For this review, take the finished solid that the model builds, in its own axes (mm). A direction names the side the tool comes from. Give positions to 0.01 mm unless a question says otherwise; leave off trailing zeros. Write each loop counter-clockwise with the first axis right and the second up, starting at its lowest first coordinate (ties: lowest second). Pieces come first, ordered by that corner, then holes.
from build123d import *

# Parameters (mm, degrees)
SKETCH1_W                = 50
SKETCH1_H                = 50
BOSS_EXTRUDE1_DEPTH      = 50
CHAMFER1_SIZE            = 1.5
BOSS_EXTRUDE2_DEPTH      = 7
BOSS_EXTRUDE2_DEPTH_BACK = 7
SKETCH6_W                = 1
SKETCH6_H                = 7
SKETCH7_W                = 1.8
SKETCH7_H                = 1.8
CUT_EXTRUDE1_DEPTH       = 7


with BuildPart() as part:
    # Sketch1 → Boss-Extrude1 (new body)
    with BuildSketch(Plane.XY):
        with Locations((25, 25)):
            Rectangle(SKETCH1_W, SKETCH1_H)
    extrude(amount=BOSS_EXTRUDE1_DEPTH)

    # Cut-Sweep2: sweep along a path in Sketch4
    with BuildLine(Plane.XY.offset(50)) as cut_sweep2_path:
        Line((25, 50), (25, 47))
        ThreePointArc((25, 47), (31.443650814, 31.443650814), (47, 25))
        Line((47, 25), (50, 25))
    # Sketch3 → Cut-Sweep2 (sweep, cut)
    with BuildSketch(Plane.XZ.offset(-50)):
        Polygon((29.556349186, 39), (36, 45.443650814), (36, 54.556349186), (29.556349186, 61), (20.443650814, 61), (14, 54.556349186), (14, 45.443650814), (20.443650814, 39), align=None)
    sweep(path=cut_sweep2_path.line, mode=Mode.SUBTRACT)

    # Sketch5 → Cut-Loft1 section 0
    with BuildSketch(Plane.ZY):
        with BuildLine():
            Line((24.5, 20.443650814), (24.5, 29.556349186))
            Line((24.5, 29.556349186), (18.056349186, 36))
            Line((18.056349186, 36), (8.943650814, 36))
            Line((8.943650814, 36), (2.5, 29.556349186))
            Line((2.5, 29.556349186), (2.5, 20.443650814))
            Line((2.5, 20.443650814), (8.943650814, 14))
            Line((8.943650814, 14), (18.056349186, 14))
            Line((18.056349186, 14), (24.5, 20.443650814))
        make_face()
    # Sketch2 → Cut-Loft1 section 1
    with BuildSketch(Plane.ZY.offset(-50)):
        with BuildLine():
            Line((36, 29.556349186), (29.556349186, 36))
            Line((29.556349186, 36), (20.443650814, 36))
            Line((20.443650814, 36), (14, 29.556349186))
            Line((14, 29.556349186), (14, 20.443650814))
            Line((14, 20.443650814), (20.443650814, 14))
            Line((20.443650814, 14), (29.556349186, 14))
            Line((29.556349186, 14), (36, 20.443650814))
            Line((36, 20.443650814), (36, 29.556349186))
        make_face()
    loft(mode=Mode.SUBTRACT)

    # Chamfer1
    chamfer1_edges = [part.edges().sort_by_distance(p)[0] for p in [
        (50, 7, 50),
        (43, 50, 50),
        (50, 43, 50),
        (7, 50, 50),
        (14, 48.5, 50),
        (23.665476221, 23.665476221, 50),
        (48.5, 14, 50),
        (36, 48.5, 50),
        (39.221825407, 39.221825407, 50),
        (48.5, 36, 50),
        (36, 50, 47.721825407),
        (14, 50, 47.721825407),
        (50, 36, 47.721825407),
        (50, 14, 47.721825407),
        (50, 17.221825407, 42.221825407),
        (50, 32.778174593, 42.221825407),
        (32.778174593, 50, 42.221825407),
        (17.221825407, 50, 42.221825407),
        (0, 25, 50),
        (25, 50, 0),
        (50, 25, 0),
        (25, 0, 0),
        (0, 25, 0),
        (25, 0, 50),
        (0, 50, 25),
        (50, 50, 25),
        (50, 0, 25),
        (0, 0, 25),
    ]]
    chamfer(chamfer1_edges, length=CHAMFER1_SIZE)

    # Sketch6 → Boss-Extrude2 (add, two sides: drawn at the far end of the back side and taken through both)
    with BuildSketch(Plane.XY.offset(50).offset(-BOSS_EXTRUDE2_DEPTH_BACK)):
        with Locations((0.5, 25)):
            Rectangle(SKETCH6_W, SKETCH6_H)
    extrude(amount=BOSS_EXTRUDE2_DEPTH + BOSS_EXTRUDE2_DEPTH_BACK)

    # Sketch7 → Cut-Extrude1 (cut)
    with BuildSketch(Plane(origin=(1, 0, 0), x_dir=(0, 0, -1), z_dir=(1, 0, 0))):
        with Locations((-53.6, 25)):
            Rectangle(SKETCH7_W, SKETCH7_H)
    extrude(amount=-CUT_EXTRUDE1_DEPTH, mode=Mode.SUBTRACT)


solid = part.part
(1) Tool access review of faces 1 (the flat face through (47.761, 32.733, 42.177)), 2 (the flat face through (49.3, 24.7, 0.8)), 3 (the flat face through (37, 49, 49)), 4 (the conical face through (37.378, 37.587, 42.983)): name each direction out of +Z, -Z, +X, -X, +Y, -Y from which nothing blocks a thin tool from reaching the whole face with its end or side.
(2) The part is to be moulded in two halves that separate along Y. For faces 5 (the flat face through (49.3, 6.9, 49.2)), 6 (the flat face through (49, 49, 1)), 7 (the flat face through (33, 32, 39)), say which applies: +Y half, -Y half, draft (parallel to the pull), parting line (faces both ways), or undercut.
(3) Clearance check with flat-ended pins moving along their axes: pin 1 Ø0.8 at (x, z) = (0.5, 53.5) entering from -Y; pin 2 Ø1.1 at (x, y) = (0.5, 24.5) entering from -Z; pin 3 Ø0.8 at (x, z) = (0.5, 54) entering from +Y. State where each tip first meets the part, or that it passes through.
(4) For L1, parallel to Y at x = 41, z = 26; L2, parallel to X at y = 46, z = 46; L3, parallel to Z at x = 13.5, y = 25.5 (3 decimals), list the stretches that pass through material, from the lowest coordinate up.
(5) We need section A-A (y = 5). Write out the cut boundary in (x, z), and give its area (3 significant figures).
(6) We need section B-B (z = 42). Write out the cut boundary in (x, y).
The answers:
1. face 1: +Z, +X
1. face 2: -Z, +X, +Y, -Y
1. face 3: +Z, +Y
1. face 4: +Z
2. face 5: draft
2. face 6: +Y half
2. face 7: undercut
3. pin 1: stops at y = 21.5
3. pin 2: stops at z = 0.45
3. pin 3: stops at y = 28.5
4. L1: y = 0 to 14, 36 to 50
4. L2: x = 0 to 14.02, 36.05 to 50
4. L3: z = 0 to 5.605, 27.605 to 50
5. outline: (0, 1.5) - (1.5, 0) - (48.5, 0) - (50, 1.5) - (50, 48.5) - (48.5, 50) - (1.5, 50) - (0, 48.5) - close
5. area: 2,500 mm2
6. outline: (0, 1.5) - (1.5, 0) - (48.5, 0) - (50, 1.5) - (50, 15.32) - (48.5, 17.44) - (47, 17.44) arc R29.56 cw to (17.44, 47) - (17.44, 48.5) - (15.32, 50) - (1.5, 50) - (0, 48.5) - close; (32.56, 47) arc R14.44 ccw to (47, 32.56) - (48.5, 32.56) - (50, 34.68) - (50, 48.5) - (48.5, 50) - (34.68, 50) - (32.56, 48.5) - close
